The model under review builds one solid part; all positions refer to its coordinate system, in mm. Round coordinates to 2 decimals unless told otherwise and drop trailing zeros. Order: outer loops, then holes, each group sorted by start corner. A loop starts at its lowest first (then second) coordinate and runs counter-clockwise, first axis right, second up.
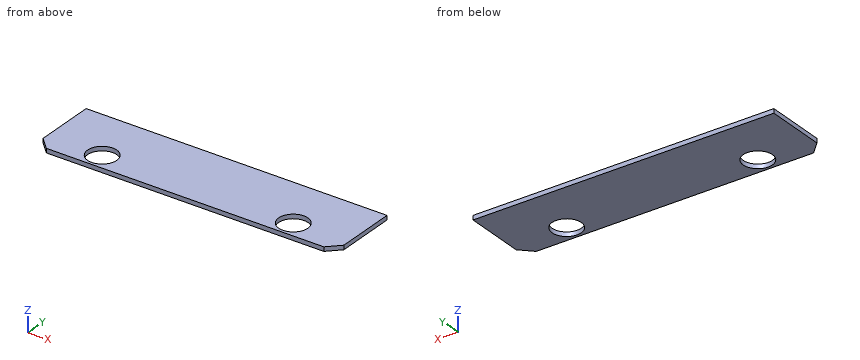
Autodesk Inventor part; units mm, degrees
ref_plane "YZ Plane" through (0, 0, 0) normal (1, 0, 0) x (0, 1, 0)
ref_plane "XZ Plane" through (0, 0, 0) normal (0, 1, 0) x (-1, 0, 0)
ref_plane "XY Plane" through (0, 0, 0) normal (0, 0, 1) x (1, 0, 0)
sketch "Sketch1" plane through (0, 0, 0) normal (0, 0, 1) x (1, 0, 0)
  line L0 (0, 0) -> (444.5, 0)
  line L1 (444.5, 0) -> (444.5, 127)
  line L2 (444.5, 127) -> (0, 127)
  line L3 (0, 127) -> (0, 0)
  dimension "d0" = 444.5
  dimension "d1" = 127
extrude "Extrusion1" add sketch "Sketch1" along normal blind 6.35
sketch "Sketch2" plane through (0, 0, 6.35) normal (0, 0, 1) x (1, 0, 0)
  line L0 (0, 0) -> (444.5, 0)
  line L1 (38.0923, 0) -> (0, 38.0919)
  line L2 (0, 127) -> (0, 0)
  line L3 (0, 0) -> (444.5, 0)
  line L4 (444.5, 0) -> (444.5, 127)
  line L5 (444.5, 0) -> (406.4, 0)
  line L6 (444.5, 0) -> (482.6, 0) construction
  line L7 (444.5, 0) -> (444.5, 38.0919)
  line L8 (444.5, 38.0919) -> (406.4086, 0)
  point P0 (419.1126, 0)
  dimension "d19" = 38.1
  dimension "d20" = 180
extrude "Extrusion2" cut sketch "Sketch2" against normal blind 50.8
sketch "Sketch3" plane through (0, 0, 6.35) normal (0, 0, 1) x (1, 0, 0)
  line L0 (0, 77.664) -> (80.645, 77.664) construction
  line L1 (444.5, 127) -> (0, 127)
  line L2 (80.645, 127) -> (161.29, 127) construction
  circle A0 centre (81.534, 46.355) radius 21.59
  line L3 (444.5, 38.0919) -> (444.5, 127)
  line L4 (444.5, 77.664) -> (525.145, 77.664) construction
  line L5 (444.5, 38.0919) -> (444.5, 127)
  line L6 (444.5, 46.355) -> (525.145, 46.355) construction
  circle A1 centre (363.855, 46.355) radius 21.59
  line L7 (444.5, 127) -> (0, 127)
  line L8 (0, 127) -> (0, 38.0919)
  circle A2 centre (58.2577, 38.8774) radius 1.8542
  circle A3 centre (58.3621, 41.6798) radius 1.8288
  circle A4 centre (104.5311, 39.3446) radius 1.8542
  circle A5 centre (104.7028, 53.3654) radius 1.8542
  point P0 (0, 0)
  dimension "d10" = 43.18
  dimension "d18" = 43.18
  dimension "d40" = 46.228
  dimension "d41" = 3.7084
  dimension "d42" = 3.6576
  dimension "d43" = 3.7084
  dimension "d44" = 3.7084
  dimension "d45" = 80.645
  dimension "d46" = 80.645
  dimension "d47" = 73.6346
  dimension "d48" = 14.0208
  dimension "d49" = 2.8024
extrude "Extrusion3" cut sketch "Sketch3" against normal blind 50.8 contours A0 | A1
thicken "Thicken1" operation add thickness 20.828 both sides no extend neighbours yes toward (0, 1, 0) faces at (160.8644, 0, 2.1167)
properties part number "MecanumDriveTrainPlate17-18"
(1) We need section A-A (x = 350.5). Give the boundary of the cut face in (y, z), and give its area (3 significant figures).
(2) We need section B-B (z = 5). Give the boundary of the cut face in (x, y) (3 decimals), and give its area (3 significant figures).
(3) We need section C-C (y = 62.5). Give the boundary of the cut face in (x, z), and give its area (3 significant figures).
(4) We need section D-D (x = 94). Give the boundary of the cut face in (y, z).
(5) To check wall thickness, follow L1, parallel to X at y = 52.5, z = 3.25; L2, parallel to X at y = 61, z = 0.5; L3, parallel to Y at x = 364, z = 1. State the ranges of each line that lie inside material, in increasing order.
Verdict:
1. outline: (20.83, 0) - (29.39, 0) - (29.39, 6.35) - (20.83, 6.35) - close; (63.32, 0) - (127, 0) - (127, 6.35) - (63.32, 6.35) - close
1. area: 459 mm2
2. outline: (0, 38.092) - (17.264, 20.828) - (427.236, 20.828) - (444.5, 38.092) - (444.5, 127) - (0, 127) - close; hole circle Ø43.18 at (81.534, 46.355); hole circle Ø43.18 at (363.855, 46.355)
2. area: 44,000 mm2
3. outline: (0, 0) - (67.2, 0) - (67.2, 6.35) - (0, 6.35) - close; (95.87, 0) - (349.52, 0) - (349.52, 6.35) - (95.87, 6.35) - close; (378.19, 0) - (444.5, 0) - (444.5, 6.35) - (378.19, 6.35) - close
3. area: 2,460 mm2
4. outline: (20.83, 0) - (28.73, 0) - (28.73, 6.35) - (20.83, 6.35) - close; (63.98, 0) - (127, 0) - (127, 6.35) - (63.98, 6.35) - close
5. L1: x = 0 to 60.84, 102.23 to 343.16, 384.55 to 444.5
5. L2: x = 0 to 65.67, 97.4 to 347.99, 379.72 to 444.5
5. L3: y = 20.83 to 24.77, 67.94 to 127
